```python
from build123d import *

# Parameters (mm, degrees)
SKETCH1_W               = 110.4
SKETCH1_H               = 110.4
SKETCH1_W_2             = 107
SKETCH1_H_2             = 107
BOSS_EXTRUDE1_DEPTH     = 2
SKETCH3_W               = 115
SKETCH3_H               = 115
BOSS_EXTRUDE2_DEPTH     = 2.3
SKETCH4_R               = 3
BOSS_EXTRUDE3_DEPTH     = 10
CUT_EXTRUDE2_DEPTH      = 82.929848041
CUT_EXTRUDE2_DEPTH_BACK = 82.929848041
SKETCH5_R               = 6.75
SKETCH5_R_2             = 6.25
SKETCH5_R_3             = 1.25
SKETCH5_W               = 7
SKETCH5_H               = 9
SKETCH5_W_2             = 34.1
SKETCH5_H_2             = 47
SKETCH5_W_3             = 28
SKETCH5_H_3             = 1
SKETCH6_R               = 1.65
BOSS_EXTRUDE4_DEPTH     = 4
SKETCH7_W               = 24.147095738
SKETCH7_H               = 14
CUT_EXTRUDE4_DEPTH      = 10
FILLET1_R               = 0.5


with BuildPart() as part:
    # Sketch1 → Boss-Extrude1 (new body)
    with BuildSketch(Plane.XY):
        Rectangle(SKETCH1_W, SKETCH1_H)
        Rectangle(SKETCH1_W_2, SKETCH1_H_2, mode=Mode.SUBTRACT)
    extrude(amount=BOSS_EXTRUDE1_DEPTH)

    # Sketch3 → Boss-Extrude2 (add)
    with BuildSketch(Plane(origin=(0, 0, 0), x_dir=(-1, 0, 0), z_dir=(0, 0, -1))):
        Rectangle(SKETCH3_W, SKETCH3_H)
    extrude(amount=BOSS_EXTRUDE2_DEPTH)

    # Sketch4 → Boss-Extrude3 (add)
    with BuildSketch(Plane.XY):
        with Locations(Location((-45.72, 45.72, 0), (0, 0, 180))):
            Circle(SKETCH4_R)
        with Locations(Location((45.72, 45.72, 0), (0, 0, 180))):
            Circle(SKETCH4_R)
        with Locations(Location((45.72, -45.72, 0), (0, 0, 180))):
            Circle(SKETCH4_R)
        with Locations(Location((-45.72, -45.72, 0), (0, 0, 180))):
            Circle(SKETCH4_R)
    extrude(amount=BOSS_EXTRUDE3_DEPTH)

    # Sketch5 → Cut-Extrude2 (cut, two sides: drawn at the far end of the back side and taken through both)
    with BuildSketch(Plane.XY.offset(-CUT_EXTRUDE2_DEPTH_BACK)):
        with Locations((-8, -28.6)):
            Circle(SKETCH5_R)
        with Locations((6.95, 31.72)):
            Circle(SKETCH5_R_2)
        with Locations((-40.75, -11)):
            Circle(SKETCH5_R_3)
        with Locations((-10.15, -11)):
            Circle(SKETCH5_R_3)
        with Locations((-10.15, 40)):
            Circle(SKETCH5_R_3)
        with Locations((-40.75, 40)):
            Circle(SKETCH5_R_3)
        with Locations((6.5, -7.2)):
            Rectangle(SKETCH5_W, SKETCH5_H)
        with Locations((-25.45, 14.5)):
            Rectangle(SKETCH5_W_2, SKETCH5_H_2)
        with Locations((-25.45, -9)):
            Rectangle(SKETCH5_W_3, SKETCH5_H_3)
    extrude(amount=CUT_EXTRUDE2_DEPTH + CUT_EXTRUDE2_DEPTH_BACK, mode=Mode.SUBTRACT)

    # Sketch6 → Boss-Extrude4 (add)
    with BuildSketch(Plane.XY.offset(10)):
        with Locations((-45.72, 45.72)):
            Circle(SKETCH6_R)
        with Locations((45.72, 45.72)):
            Circle(SKETCH6_R)
        with Locations((45.72, -45.72)):
            Circle(SKETCH6_R)
        with Locations((-45.72, -45.72)):
            Circle(SKETCH6_R)
    extrude(amount=BOSS_EXTRUDE4_DEPTH)

    # Sketch7 → Cut-Extrude4 (cut)
    with BuildSketch(Plane.XY):
        with Locations((57.5, -7.2)):
            Rectangle(SKETCH7_W, SKETCH7_H)
    extrude(amount=CUT_EXTRUDE4_DEPTH, mode=Mode.SUBTRACT)

    # Fillet1
    fillet1_edges = [part.edges().sort_by_distance(p)[0] for p in [
        (-11.45, -9.5, -1.15),
        (-39.45, -9.5, -1.15),
    ]]
    fillet(fillet1_edges, radius=FILLET1_R - 0.0001)  # a hair under: the kernel refuses the full size


solid = part.part
```
Design review of the part built by this model. Coordinates are the model's own, in mm. A direction names the side the tool comes from. Coordinates: 2 decimals unless noted, no trailing zeros. Write each loop counter-clockwise with the first axis right and the second up, starting at its lowest first coordinate (ties: lowest second). Pieces come first, ordered by that corner, then holes. Notation, with made-up numbers: M 11.25,-9 L 59.25,-9 A13 cw 59.25,-2 Z; hole C -20.75,-40 d6. An arc over 180 degrees is marked long. Answer as a JSON object with one key per item and string values.
Item 1: Add section C-C, the plane x = -45.72. Give the boundary of the cut face in (y, z).
Outcome:
{"outline": "M -57.5,-2.3 L 57.5,-2.3 L 57.5,0 L 55.2,0 L 55.2,2 L 53.5,2 L 53.5,0 L 48.72,0 L 48.72,10 L 47.37,10 L 47.37,14 L 44.07,14 L 44.07,10 L 42.72,10 L 42.72,0 L -42.72,0 L -42.72,10 L -44.07,10 L -44.07,14 L -47.37,14 L -47.37,10 L -48.72,10 L -48.72,0 L -53.5,0 L -53.5,2 L -55.2,2 L -55.2,0 L -57.5,0 Z"}
Item 2: Insertion check: pin 1 Ø1.6 at (x, z) = (-10, 1) entering from +Y; pin 2 Ø6 at (x, y) = (-6.5, 27) entering from +Z; pin 3 Ø1.6 at (y, z) = (-41.5, 1) entering from +X. Each pin has a flat end and moves straight along its axis. Give the tip position at first contact, or say it passes through.
Outcome:
{"pin 1": "y = 55.2", "pin 2": "z = 0", "pin 3": "x = 55.2"}
Item 3: Draft analysis for pull direction X (two halves, no side actions). For faces 1 (the cylindrical face through (-48.58, 44.82, 4.93)), 2 (the flat face through (-46, 46, 14)), state which applies: pulls with the +X half, pulls with the -X half, needs draft (parallel to the pull), parting line crosses it, or undercut.
Outcome:
{"face 1": "undercut", "face 2": "needs draft"}
Item 4: Add section B-B, the plane y = 31.72. Give the boundary of the cut face in (x, z), and give its area (3 significant figures).
Outcome:
{"outline": "M -57.5,-2.3 L -42.5,-2.3 L -42.5,0 L -53.5,0 L -53.5,2 L -55.2,2 L -55.2,0 L -57.5,0 Z; M -8.4,-2.3 L 0.7,-2.3 L 0.7,0 L -8.4,0 Z; M 13.2,-2.3 L 57.5,-2.3 L 57.5,0 L 55.2,0 L 55.2,2 L 53.5,2 L 53.5,0 L 13.2,0 Z", "area": "164 mm²"}
Item 5: Add section D-D, the plane z = 7.25. Give the boundary of the cut face in (x, y).
Outcome:
{"outline": "C -45.72,-45.72 d6; C -45.72,45.72 d6; C 45.72,-45.72 d6; C 45.72,45.72 d6"}
Item 6: Wall thickness on probe 1 along Y at (x, z) = (-40.75, -1.5); probe 2 along Y at (x, z) = (6.95, -1.7); probe 3 along X at (y, z) = (-11, -1.1): over which ranges is each line inside the solid? List them lowest first.
Outcome:
{"probe 1": "-57.5 to -12.25, -9.75 to -9, 38 to 38.75, 41.25 to 57.5", "probe 2": "-57.5 to -11.7, -2.7 to 25.47, 37.97 to 57.5", "probe 3": "-57.5 to -42, -39.5 to -11.4, -8.9 to 3, 10 to 57.5"}
Item 7: Machinability: for faces 3 (the cylindrical face through (-1.765, -31.185, -1.166)), 4 (the flat face through (44, -44, 10)), which of the approach directions +Z, -Z, +X, -X, +Y, -Y give a long, thin tool a straight path to every point of the face, cutting with its end or side? Answer none if there is none.
Outcome:
{"face 3": "+Z, -Z", "face 4": "+Z"}
Item 8: Add section A-A, the plane x = -27. Give the boundary of the cut face in (y, z).
Outcome:
{"outline": "M -57.5,-2.3 L -9.5,-2.3 L -9.5,0 L -53.5,0 L -53.5,2 L -55.2,2 L -55.2,0 L -57.5,0 Z; M 38,-2.3 L 57.5,-2.3 L 57.5,0 L 55.2,0 L 55.2,2 L 53.5,2 L 53.5,0 L 38,0 Z"}
